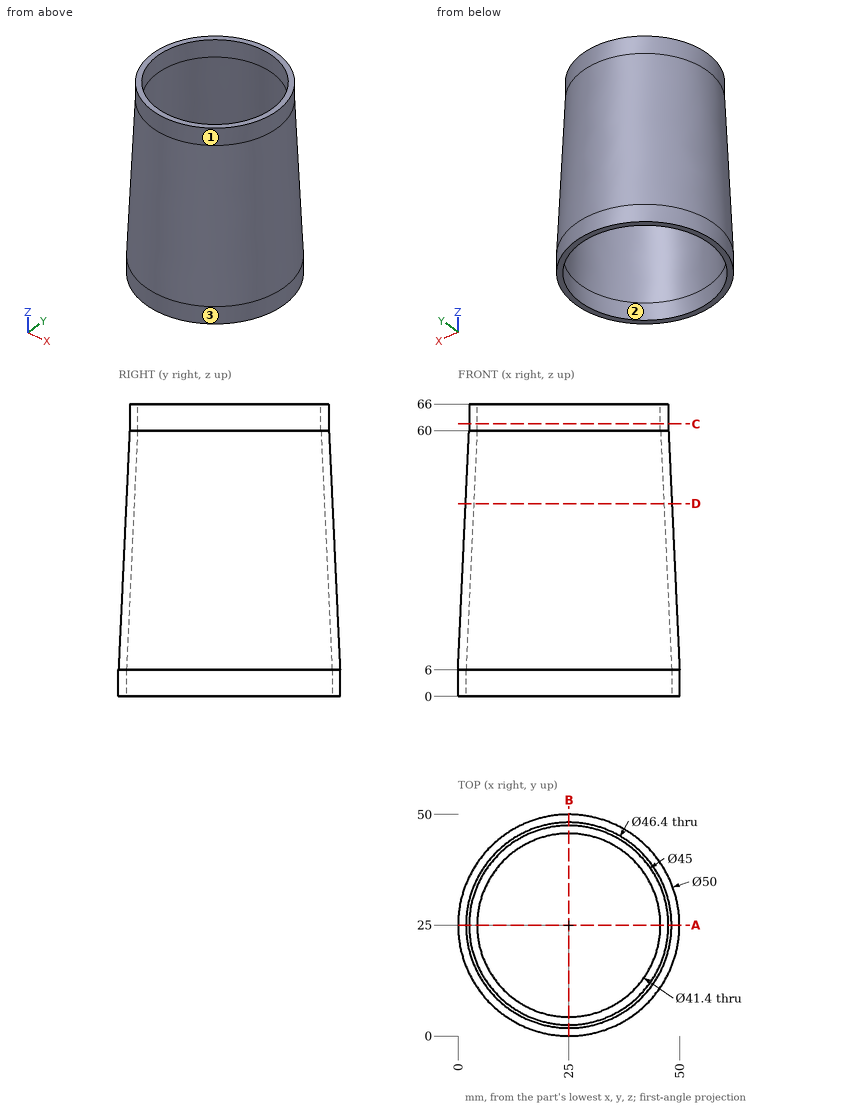
Can you work these out from the drawing? Everything is in mm from the part's minimum corner. A direction names the side the tool comes from. Give positions to 0.01 mm unless a question says otherwise; leave off trailing zeros. Loops run counter-clockwise (first coordinate to the right, second up) from the corner with the lowest first, then second, coordinate; pieces in that order, holes last. Notation, with made-up numbers: M -28,-7 L 9,-7 A26 ccw 9,15 Z; hole C 15,11.5 d1. An arc over 180 degrees is marked long. Use CSV: the item, a comma, the result in double quotes. Start each with the question number.
1. Imagine slicing it at C-C, the plane z = 61.5. Write out the boundary of the cut face in (x, y).
2. If I drill on L1, parallel to Y at x = 25, z = 63; L2, parallel to Y at x = 25, z = 2, over which ranges is the centre line in solid material (lowest first)?
3. On a 3-axis mill with a long thin cutter (end or side, diameter ignored), from which of +Z, -Z, +X, -X, +Y, -Y can I reach the whole of each face in a straight line? I mean the marked faces 1, 2 and 3. Say none if no direction works.
4. Imagine slicing it at A-A, the plane y = 25. Write out the boundary of the cut face in (x, z), plus the area to 3 significant figures.
5. For P1, Ø10, axis at x = 30.5, z = 15.5, coming from the +Y side; P2, Ø3, axis at x = 8.5, y = 17, coming from the +Z side; P3, Ø5, axis at y = 12, z = 37.5, coming from the +X side; P4, Ø6, axis at y = 6.5, z = 28, coming from the +X side, each with a flat end and sliding along its axis, tell me the tip position at first contact or that it passes through.
6. Imagine slicing it at D-D, the plane z = 43.5. Write out the boundary of the cut face in (x, y).
Response values:
1,outline,"C 25,25 d45; hole C 25,25 d41.4"
2,L1,"2.5 to 4.3, 45.7 to 47.5"
2,L2,"0 to 1.8, 48.2 to 50"
3,face 1,"+Z"
3,face 2,"-Z"
3,face 3,"+Z, -Z"
4,outline,"M 0,0 L 1.8,0 L 1.8,6 L 4.3,60 L 4.3,66 L 2.5,66 L 2.5,60 L 0,6 Z; M 45.7,60 L 48.2,6 L 48.2,0 L 50,0 L 50,6 L 47.5,60 L 47.5,66 L 45.7,66 Z"
4,area,"238 mm^2"
5,P1,"y = 49.65"
5,P2,"through"
5,P3,"x = 46.08"
5,P4,"x = 43.31"
6,outline,"C 25,25 d46.53; hole C 25,25 d42.93"
